Input: part model. Units: mm. Frame: model coordinates. Face numbers are marked on the shaded views. A direction names the side the tool comes from. Give positions to 0.01 mm unless a question says otherwise; leave off trailing zeros. Loops run counter-clockwise (first coordinate to the right, second up) from the corner with the lowest first, then second, coordinate; pieces in that order, holes last. Notation, with made-up numbers: M -32,-14.5 L 20,-14.5 A12 cw 20,-2.5 Z; hole C 26.25,85 d10. An arc over 180 degrees is marked long. Use CSV: the item, a comma, the result in double quotes. Start each with the question number.
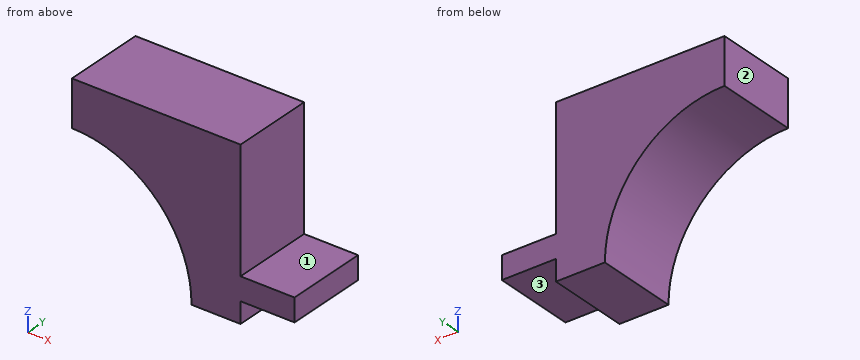
from build123d import *

# Parameters (mm, degrees)
BOSS_EXTRUDE1_DEPTH = 18


with BuildPart() as part:
    # Sketch1 → Boss-Extrude1 (new body)
    with BuildSketch(Plane(origin=(0, 0, 0), x_dir=(1, 0, 0), z_dir=(0, 1, 0))):
        with BuildLine():
            Line((-24, 305), (-13.36, 305))
            Line((-13.36, 305), (-13.36, 300.43))
            Line((-13.36, 300.43), (-1.616090732, 300.43))
            Line((-1.616090732, 300.43), (-1.616090732, 295.43))
            Line((-1.616090732, 295.43), (-13.36, 295.43))
            Line((-13.36, 295.43), (-13.36, 269))
            Line((-13.36, 269), (-50, 269))
            Line((-50, 269), (-50, 279))
            ThreePointArc((-50, 279), (-31.615223689, 286.615223689), (-24, 305))
        make_face()
    extrude(amount=BOSS_EXTRUDE1_DEPTH)


solid = part.part
Item 1: Material intervals for line 1 (Z direction, x = -6, y = 1.5); line 2 (X direction, y = 10.25, z = -271); line 3 (X direction, y = 7, z = -302.5), sorted ascending.
Item 2: First-contact query: pin 1 Ø9.5 at (x, y) = (-8.5, 8) entering from +Z; pin 2 Ø3.5 at (y, z) = (9, -302.5) entering from +X. Flat tips, straight axial feed; report the tip coordinate or a pass-through.
Item 3: Section C-C (x = -39.5). Output: boundary loops of the cut face in (y, z), then the cut area to 3 significant figures.
Item 4: Set-up query: the marked faces 1, 2 and 3. Return all of +Z, -Z, +X, -X, +Y, -Y with unobstructed straight access to the full face (end or side cutting, diameter ignored); none if empty.
Item 5: Section A-A (y = 2.25). Output: boundary loops of the cut face in (x, z).
Item 6: Section B-B (z = -278). Output: boundary loops of the cut face in (x, y).
Recorded:
1,line 1,"-300.43 to -295.43"
1,line 2,"-50 to -13.36"
1,line 3,"-24.12 to -13.36"
2,pin 1,"z = -295.43"
2,pin 2,"x = -13.36"
3,outline,"M 0,-281.21 L 18,-281.21 L 18,-269 L 0,-269 Z"
3,area,"220 mm²"
4,face 1,"+Z, +X, +Y, -Y"
4,face 2,"+Z, -Z, -X, +Y, -Y"
4,face 3,"-Z, +X, +Y, -Y"
5,outline,"M -50,-279 A26 cw -24,-305 L -13.36,-305 L -13.36,-300.43 L -1.62,-300.43 L -1.62,-295.43 L -13.36,-295.43 L -13.36,-269 L -50,-269 Z"
6,outline,"M -50,0 L -13.36,0 L -13.36,18 L -50,18 Z"
